Read the model definition and answer for the solid it produces. Units are mm, in the model's axes. A direction names the side the tool comes from. Coordinates: 2 decimals unless noted, no trailing zeros. Order: outer loops, then holes, each group sorted by start corner. A loop starts at its lowest first (then second) coordinate and runs counter-clockwise, first axis right, second up. Notation, with made-up numbers: M -14,35.25 L 37,35.25 A11 ccw 37,51.25 Z; hole C 62.25,-25.5 d9. An arc over 180 degrees is marked long. One line per question, with ' | ' between items. Start each with the question number.
1) A tool of negligible diameter and unlimited length cuts with its end or side. For faces 1 (the face through (286, -25, 69)), 2 (the face through (140.998, -10.955, -83.434)), from which of +Z, -Z, +X, -X, +Y, -Y can it reach the whole face along a straight path? Write none if from no direction.
2) Find section C-C, the plane x = 39. Write down the section's boundary in (y, z), plus the area to 3 significant figures.
3) Given P1, Ø5, axis at y = 44.5, z = 105, coming from the -X side; P2, Ø10, axis at y = -32, z = 96.5, coming from the +X side; P3, Ø4, axis at x = 45.5, z = -14.5, coming from the +Y side, each flat-ended and moving along its own axis, determine where each tip first touches the part or whether it passes through.
4) Find section A-A, the plane z = 0. Write down the section's boundary in (x, y), plus the area to 3 significant figures.
5) Find section B-B, the plane y = 0. Write down the section's boundary in (x, z).
6) Find section D-D, the plane z = 102. Write down the section's boundary in (x, y), plus the area to 3 significant figures.
7) Consider probe 1 along Z at (x, y) = (259, 3); probe 2 along Z at (x, y) = (256, 6); probe 3 along Y at (x, z) = (36.5, -21). Determine where each line is inside the solid, lowest interval first.
8) The mould has two halves that part along X. Classify faces 3 (the face through (141, 3.22, -73.08)), 4 (the face through (180.55, -58.9, 101.34)), 5 (the face through (83.208, 2.631, 100.74)), 6 (the face through (0, -25, 69)): +X half, -X half, draft (parallel to the pull), parting line (faces both ways), or undercut.
Autodesk Inventor part; units mm, degrees
ref_plane "YZ Plane" through (0, 0, 0) normal (1, 0, 0) x (0, 1, 0)
ref_plane "XZ Plane" through (0, 0, 0) normal (0, 1, 0) x (-1, 0, 0)
ref_plane "XY Plane" through (0, 0, 0) normal (0, 0, 1) x (1, 0, 0)
sketch "Sketch1" plane through (0, 0, 0) normal (1, 0, 0) x (0, 1, 0)
  circle A0 centre (0, 0) radius 84.15
  dimension "d0" = 168.3
extrude "Extrude1" add sketch "Sketch1" along normal blind 286
sketch "Sketch2" plane through (0, 0, 0) normal (0, 0, 1) x (1, 0, 0)
  line L0 (0, 84.15) -> (0, -84.15)
  line L1 (286, 84.15) -> (286, -84.15)
  line L2 (0, 0) -> (286, 0) construction
  circle A0 centre (143, 0) radius 69.85
  dimension "d3" = 139.7
extrude "Extrude2" add sketch "Sketch2" along normal blind 137
sketch "Sketch3" plane through (0, 0, 0) normal (-1, 0, 0) x (0, 0, 1)
  circle A0 centre (0, 0) radius 84.15
  circle A1 centre (0, 0) radius 73.15
  dimension "a" = 143
  dimension "d6" = 146.3
extrude "Extrude3" cut sketch "Sketch3" against normal through all contours A1
sketch "Sketch4" plane through (143, 0, 137) normal (0, 0, 1) x (1, 0, 0)
  circle A0 centre (0, 0) radius 69.85
  circle A1 centre (0, 0) radius 59.85
  dimension "d9" = 119.7
extrude "Extrude4" cut sketch "Sketch4" against normal up to next contours A1
equation "\"d0\" = D1"
equation "\"d1\" = 2 * a"
equation "\"d3\" = D2"
equation "\"d4\" = b"
equation "\"a\" = 143"
equation "\"d6\" = D1 - 2 * s1"
equation "\"d7\" = a"
equation "\"d9\" = D2 - 2 * s2"
equation "\"d10\" = a"
equation "\"D1\" = 168.3"
equation "\"s1\" = 11"
equation "\"D2\" = 139.7"
equation "\"b\" = 137"
equation "\"Size_Designation\" = 1.2345"
properties part number "DIN 2615-1 Reducing Tee 168.3 x 11 - 139.7 x 10 S" material "Steel"
Report:
1) face 1: +Z, -Z, +X, +Y, -Y | face 2: none
2) outline: C 0,0 d168.3; hole C 0,0 d146.3 | area: 5,440 mm^2
3) P1: stops at x = 87.19 | P2: stops at x = 207.42 | P3: stops at y = 83.22
4) outline: M 0,-84.15 L 286,-84.15 L 286,-73.15 L 0,-73.15 Z; M 0,73.15 L 286,73.15 L 286,84.15 L 0,84.15 Z | area: 6,290 mm^2
5) outline: M 0,-84.15 L 286,-84.15 L 286,-73.15 L 0,-73.15 Z; M 0,73.15 L 83.15,73.15 L 83.15,137 L 73.15,137 L 73.15,84.15 L 0,84.15 Z; M 202.85,73.15 L 286,73.15 L 286,84.15 L 212.85,84.15 L 212.85,137 L 202.85,137 Z
6) outline: C 143,0 d139.7; hole C 143,0 d119.7 | area: 4,070 mm^2
7) probe 1: z = -84.1 to -73.09, 73.09 to 84.1 | probe 2: z = -83.94 to -72.9, 72.9 to 83.94 | probe 3: y = -81.49 to -70.07, 70.07 to 81.49
8) face 3: draft | face 4: parting line | face 5: undercut | face 6: -X half
